Source: CAD feature listing. Evaluate the final solid. Frame: model axes, mm. A direction names the side the tool comes from. Round coordinates to 2 decimals unless told otherwise and drop trailing zeros. Loops run counter-clockwise (first coordinate to the right, second up) from the corner with the lowest first, then second, coordinate; pieces in that order, holes last.
Item 1: Access query for faces 1 (the flat face through (-1, 127, 1)), 2 (the flat face through (-1, 64, -60.325)). Directions: +Z, -Z, +X, -X, +Y, -Y. A direction counts if a zero-diameter tool reaches every point of the face in a straight line with its end or side. Return the directions, or none.
Item 2: Pull-direction query (X, two-part tool) for faces 3 (the flat face through (63.5, 63, -57)), 4 (the flat face through (-1, 63, -63.5)), 5 (the flat face through (-61.912, 8, 2)); classes: released by +X, released by -X, zero draft, split by the parting line, or undercut.
Item 3: First-contact query: P1, Ø1.5, axis at x = 7, y = 45.5, coming from the +Z side (3 decimals); P2, Ø1.7, axis at x = -62.5, z = -2.5, coming from the -Y side. Flat tips, straight axial feed; report the tip coordinate or a pass-through.
Item 4: Section query B-B on z = -24. Return loops of the section in (x, y), then the cut area to 4 significant figures.
Item 5: Section query A-A on y = 96.5. Return loops of the section in (x, z) (1 decimal), then the cut area to 3 significant figures.
Item 6: Section query C-C on x = 31. Return loops of the section in (y, z) (1 decimal), then the cut area to 3 significant figures.
Item 7: Ray query, L1, parallel to Y at x = -53, z = 19; L2, parallel to X at y = 48, z = 57; L3, parallel to Y at x = -22, z = -42.5. Return the intervals inside material, ascending.
```python
from build123d import *

# Parameters (mm, degrees)
F0_W     = 127
F0_H     = 127
F1_DEPTH = 127
F2_W     = 101.6
F2_H     = 101.6
F3_DEPTH = 123.825
F4_W     = 101.6
F4_H     = 101.6
F5_DEPTH = 127.001
F6_W     = 123.825
F6_H     = 123.825
F7_DEPTH = 123.825


with BuildPart() as f1:
    # F0 (on Front) → F1 (new body)
    with BuildSketch(Plane.XZ):
        Rectangle(F0_W, F0_H)
    extrude(amount=-F1_DEPTH)

    # F2 (on face) → F3 (cut)
    with BuildSketch(Plane.XZ):
        with Locations((0, -1.39066)):
            Rectangle(F2_W, F2_H)
    extrude(amount=-F3_DEPTH, mode=Mode.SUBTRACT)

    # F4 (on face) → F5 (cut, through all)
    with BuildSketch(Plane.YZ.offset(63.5)):
        with Locations((63.5, 0)):
            Rectangle(F4_W, F4_H)
    extrude(amount=-F5_DEPTH, mode=Mode.SUBTRACT)

    # F6 (on face) → F7 (cut)
    with BuildSketch(Plane.XY.offset(63.5)):
        with Locations((0, 63.5)):
            Rectangle(F6_W, F6_H)
    extrude(amount=-F7_DEPTH, mode=Mode.SUBTRACT)


solid = f1.part
```
Data:
1. face 1: +Z, -Z, +X, -X, +Y
1. face 2: +Z
2. face 3: released by +X
2. face 4: zero draft
2. face 5: undercut
3. P1: stops at z = -60.325
3. P2: stops at y = 0
4. outline: (-63.5, 0) - (-50.8, 0) - (-50.8, 1.59) - (-61.91, 1.59) - (-61.91, 12.7) - (-63.5, 12.7) - close; (-63.5, 114.3) - (-61.91, 114.3) - (-61.91, 125.41) - (61.91, 125.41) - (61.91, 114.3) - (63.5, 114.3) - (63.5, 127) - (-63.5, 127) - close; (50.8, 0) - (63.5, 0) - (63.5, 12.7) - (61.91, 12.7) - (61.91, 1.59) - (50.8, 1.59) - close
4. area: 312.5 mm2
5. outline: (-63.5, -63.5) - (63.5, -63.5) - (63.5, -50.8) - (61.9, -50.8) - (61.9, -60.3) - (-61.9, -60.3) - (-61.9, -50.8) - (-63.5, -50.8) - close; (-63.5, 50.8) - (-61.9, 50.8) - (-61.9, 63.5) - (-63.5, 63.5) - close; (61.9, 50.8) - (63.5, 50.8) - (63.5, 63.5) - (61.9, 63.5) - close
5. area: 474 mm2
6. outline: (0, -63.5) - (127, -63.5) - (127, 63.5) - (125.4, 63.5) - (125.4, -60.3) - (1.6, -60.3) - (1.6, -52.2) - (0, -52.2) - close; (0, 49.4) - (1.6, 49.4) - (1.6, 63.5) - (0, 63.5) - close
6. area: 635 mm2
7. L1: y = 0 to 1.59, 125.41 to 127
7. L2: x = -63.5 to -61.91, 61.91 to 63.5
7. L3: y = 125.41 to 127
